Check sheet for the modelled part. Datum: model origin and axes. Units: mm. A direction names the side the tool comes from. Round coordinates to 2 decimals unless told otherwise and drop trailing zeros. Write each loop counter-clockwise with the first axis right and the second up, starting at its lowest first coordinate (ties: lowest second). Pieces come first, ordered by that corner, then holes.
Item 1: Cross-section at A-A on y = 0. Enter the section's corners in (x, z), plus the area to 3 significant figures.
Item 2: Go/stop test with flat-tipped pins: pin 1 Ø3.5 at (x, y) = (-5.5, 0) entering from -Z; pin 2 Ø3 at (y, z) = (4.5, 51) entering from +X; pin 3 Ø4 at (x, z) = (1.5, 10.5) entering from +Y; pin 4 Ø1 at (y, z) = (-1, 33.5) entering from -X. Record where each tip stops, or that it passes through.
Item 3: Cross-section at C-C on z = 10. Enter the section's corners in (x, y).
Item 4: Cross-section at D-D on x = -5.5. Enter the section's corners in (y, z).
Item 5: Cross-section at B-B on x = 0. Enter the section's corners in (y, z), plus the area to 3 significant figures.
Item 6: Release check for a two-part mould opening along X. For faces 4 (the cylindrical face through (-0.325, -1.464, 62.234)), 5 (the flat face through (-6, 0, 37.5)), 6 (the flat face through (0, -6.928, 16)) record: +X half, -X half, draft (parallel to the pull), parting line (faces both ways), or undercut.
Item 7: Material ranges on line 1 (X direction, y = 0.75, z = 42); line 2 (Z direction, x = -0.5, y = 6.75); line 3 (Z direction, x = -1.75, y = 7), recorded low to high.
Item 8: Tool access check on faces 1 (the cylindrical face through (-6.59, 0.05, 40.54)), 2 (the flat face through (0, 6.928, 16)), 3 (the flat face through (0, 1.218, 66)). Record the directions out of +Z, -Z, +X, -X, +Y, -Y that give a thin tool (end or side, any length) a straight path to the whole face; none if there is none.
from build123d import *

# Parameters (mm, degrees)
SKETCH1_R           = 8
BOSS_EXTRUDE1_DEPTH = 32
CUT_EXTRUDE1_DEPTH  = 32
SKETCH4_R           = 8
BOSS_EXTRUDE2_DEPTH = 11.5
SKETCH5_R           = 1.0922
CUT_EXTRUDE2_DEPTH  = 6
SKETCH5_3_R         = 1.5
BOSS_EXTRUDE3_DEPTH = 38
CUT_EXTRUDE3_START  = -30
CUT_EXTRUDE3_DEPTH  = 30


with BuildPart() as part:
    # Sketch1 → Boss-Extrude1 (new body)
    with BuildSketch(Plane.XY):
        Circle(SKETCH1_R)
    extrude(amount=BOSS_EXTRUDE1_DEPTH)

    # Sketch3 → Cut-Extrude1 (cut)
    with BuildSketch(Plane(origin=(0, 0, 0), x_dir=(-1, 0, 0), z_dir=(0, 0, -1))):
        with BuildLine():
            ThreePointArc((4, 6.92820323), (0, 8), (-4, 6.92820323))
            Line((-4, 6.92820323), (4, 6.92820323))
        make_face()
        with BuildLine():
            Line((4, -6.92820323), (-4, -6.92820323))
            ThreePointArc((-4, -6.92820323), (0, -8), (4, -6.92820323))
        make_face()
    extrude(amount=-CUT_EXTRUDE1_DEPTH, mode=Mode.SUBTRACT)

    # Sketch4 → Boss-Extrude2 (add)
    with BuildSketch(Plane.XY.offset(32)):
        with Locations(Location((0, 0, 0), (0, 0, 120))):
            Circle(SKETCH4_R)
    extrude(amount=BOSS_EXTRUDE2_DEPTH)

    # Sketch5 → Cut-Extrude2 (cut)
    with BuildSketch(Plane.XY.offset(43.5)):
        with Locations((-5.5, 0)):
            Circle(SKETCH5_R)
        with Locations((5.5, 0)):
            Circle(SKETCH5_R)
    extrude(amount=-CUT_EXTRUDE2_DEPTH, mode=Mode.SUBTRACT)

    # Sketch5_3 → Boss-Extrude3 (add)
    with BuildSketch(Plane.XY.offset(43.5)):
        Circle(SKETCH5_3_R)
    extrude(amount=BOSS_EXTRUDE3_DEPTH)

    # Sketch6 → Cut-Extrude3 (cut)
    with BuildSketch(Plane.XY.offset(81.5).offset(CUT_EXTRUDE3_START)):
        with BuildLine():
            Line((-0.875, 1.218349293), (0.875, 1.218349293))
            ThreePointArc((0.875, 1.218349293), (0, 1.5), (-0.875, 1.218349293))
        make_face()
    extrude(amount=CUT_EXTRUDE3_DEPTH, mode=Mode.SUBTRACT)


solid = part.part
Response values:
1. outline: (-8, 0) - (8, 0) - (8, 43.5) - (6.59, 43.5) - (6.59, 37.5) - (4.41, 37.5) - (4.41, 43.5) - (1.5, 43.5) - (1.5, 81.5) - (-1.5, 81.5) - (-1.5, 43.5) - (-4.41, 43.5) - (-4.41, 37.5) - (-6.59, 37.5) - (-6.59, 43.5) - (-8, 43.5) - close
1. area: 784 mm2
2. pin 1: stops at z = 0
2. pin 2: passes through
2. pin 3: stops at y = 6.93
2. pin 4: stops at x = -7.98
3. outline: (-4, -6.93) - (4, -6.93) arc R8 ccw to (4, 6.93) - (-4, 6.93) arc R8 ccw to start
4. outline: (-5.81, 0) - (5.81, 0) - (5.81, 43.5) - (1.09, 43.5) - (1.09, 37.5) - (-1.09, 37.5) - (-1.09, 43.5) - (-5.81, 43.5) - close
5. outline: (-8, 32) - (-6.93, 32) - (-6.93, 0) - (6.93, 0) - (6.93, 32) - (8, 32) - (8, 43.5) - (1.5, 43.5) - (1.5, 51.5) - (1.22, 51.5) - (1.22, 81.5) - (-1.5, 81.5) - (-1.5, 43.5) - (-8, 43.5) - close
5. area: 733 mm2
6. face 4: parting line
6. face 5: undercut
6. face 6: draft
7. line 1: x = -7.96 to -6.29, -4.71 to 4.71, 6.29 to 7.96
7. line 2: z = 0 to 43.5
7. line 3: z = 32 to 43.5
8. face 1: +Z
8. face 2: -Z, +X, -X, +Y
8. face 3: +Z, +X, -X, +Y
